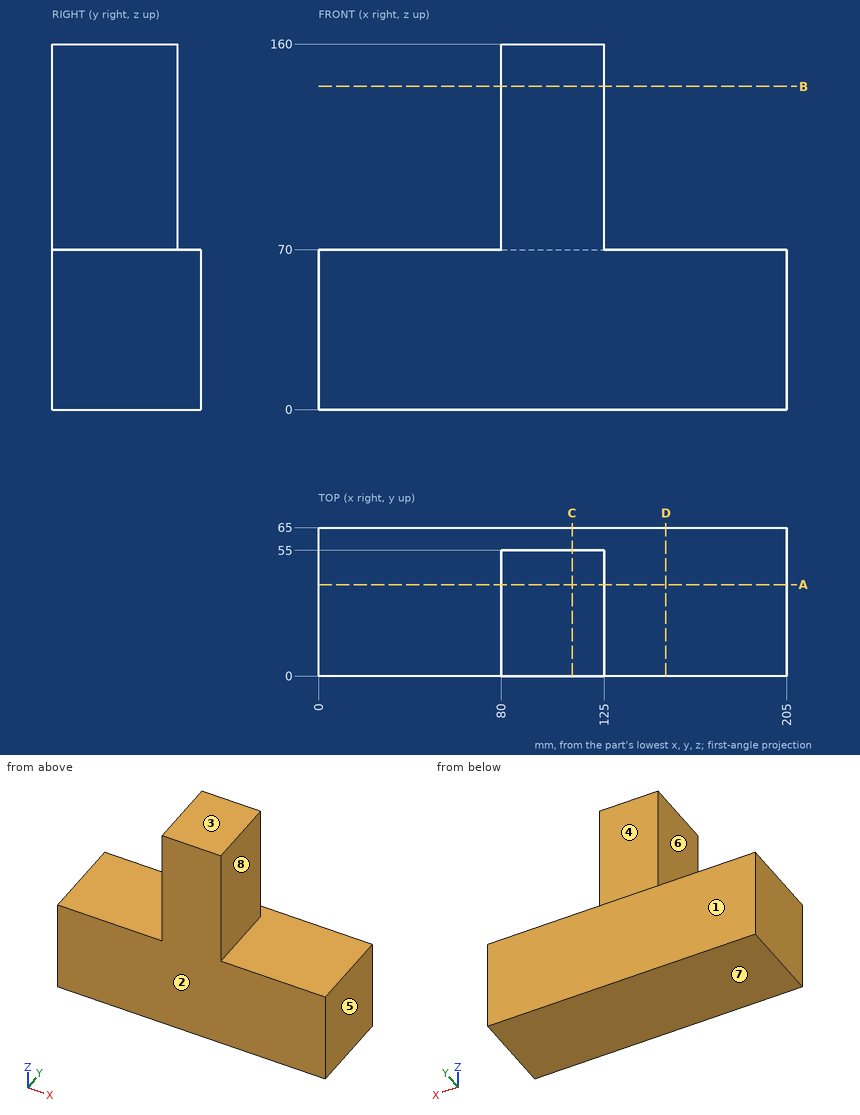
Study the drawing (mm; zero at the part's minimum x, y, z) and answer. A direction names the side the tool comes from. Give positions to 0.01 mm unless a question says otherwise; leave off trailing zeros. Loops run counter-clockwise (first coordinate to the right, second up) from the corner with the lowest first, then second, coordinate; pieces in that order, holes last. Notation, with made-up numbers: (56, 4.5) -> (114, 4.5) arc R24 ccw to (114, 29.5) -> close; hole circle Ø4 at (-21.5, 42.25). An arc over 180 degrees is marked (long way). Use a Markdown table: item, result. Add a question column.
1) The part is cut by section A-A, the plane y = 40. Determine the outline of the cut face in (x, z), plus the area to 3 significant figures.
2) The part is cut by section C-C, the plane x = 111. Determine the outline of the cut face in (y, z).
3) Which of the six approach directions +Z, -Z, +X, -X, +Y, -Y give full straight-line access (tool end or side, diameter ignored) to the marked faces 4, 5, 6, 7 and 8?
4) Each of these flat-tipped pins is pushed along its axis until it touches: P1, Ø5, axis at x = 162.5, y = 55, coming from the +Z side; P2, Ø2, axis at y = 57.5, z = 125, coming from the -X side; P3, Ø1, axis at y = 34, z = 82.5, coming from the +X side. Where does it stop, or does it pass through?
5) For a pull along Y with two mould halves and no side action, classify the marked faces 1, 2 and 3 as +Y half, -Y half, draft (parallel to the pull), parting line (faces both ways), or undercut.
6) The part is cut by section D-D, the plane x = 152. Determine the outline of the cut face in (y, z).
7) Consider line 1 along X through (y, z) = (42, 152); line 2 along Z through (x, y) = (72, 61). Determine where each line is inside the solid, lowest interval first.
8) The part is cut by section B-B, the plane z = 141.5. Determine the outline of the cut face in (x, y), plus the area to 4 significant figures.
Reported:
| question | item | result |
|---|---|---|
| 1 | outline | (0, 0) -> (205, 0) -> (205, 70) -> (125, 70) -> (125, 160) -> (80, 160) -> (80, 70) -> (0, 70) -> close |
| 1 | area | 18,400 mm^2 |
| 2 | outline | (0, 0) -> (65, 0) -> (65, 70) -> (55, 70) -> (55, 160) -> (0, 160) -> close |
| 3 | face 4 | +Z, +X, -X, +Y |
| 3 | face 5 | +Z, -Z, +X, +Y, -Y |
| 3 | face 6 | +Z, -X, +Y, -Y |
| 3 | face 7 | -Z, +X, -X, +Y, -Y |
| 3 | face 8 | +Z, +X, +Y, -Y |
| 4 | P1 | stops at z = 70 |
| 4 | P2 | passes through |
| 4 | P3 | stops at x = 125 |
| 5 | face 1 | +Y half |
| 5 | face 2 | -Y half |
| 5 | face 3 | draft |
| 6 | outline | (0, 0) -> (65, 0) -> (65, 70) -> (0, 70) -> close |
| 7 | line 1 | x = 80 to 125 |
| 7 | line 2 | z = 0 to 70 |
| 8 | outline | (80, 0) -> (125, 0) -> (125, 55) -> (80, 55) -> close |
| 8 | area | 2,475 mm^2 |
